Autodesk Fusion 360 part; units mm, degrees
sketch "Sketch1" plane through (0, 0, 0) normal (0, 0, 1) x (1, 0, 0)
  line L0 (33, 21) -> (-33, 21)
  line L1 (-33, 21) -> (-33, -21)
  line L2 (-33, -21) -> (33, -21)
  line L3 (33, -21) -> (33, 21)
  line L4 (33, 21) -> (-33, -21) construction
  line L5 (-33, 21) -> (33, -21) construction
  dimension "d1" = 66
  dimension "d2" = 42
extrude "Extrude1" add sketch "Sketch1" along normal blind 12
chamfer "Chamfer1" distance 12 angle 45 2 edges at (33, -21, 6) (33, 21, 6)
sketch "Sketch2" plane through (0, 0, 12) normal (0, 0, 1) x (-1, 0, 0)
  line L0 (-33, -9) -> (-21, -21)
  line L1 (-21, -21) -> (33, -21)
  line L2 (33, -21) -> (33, 21)
  line L3 (33, 21) -> (-21, 21)
  line L4 (-21, 21) -> (-33, 9)
  line L5 (-33, 9) -> (-33, -9)
  line L6 (33, -21) -> (21, -21)
  line L7 (21, -21) -> (21, 21)
  line L8 (21, 21) -> (33, 21)
  line L9 (33, 21) -> (33, -21)
  dimension "d6" = 12
extrude "Extrude2" add sketch "Sketch2" along normal blind 48 contours L1 L2 L3 L6 L7 L8 L9
fillet "Fillet1" radius 21 2 edges at (-27, 21, 60) (-27, -21, 60)
sketch "Sketch3" plane through (0, 0, 0) normal (0, 1, 0) x (1, 0, 0)
  line L0 (-20.8442, -53.799) -> (-20.8442, -11.799)
  line L1 (-20.8442, -11.799) -> (33.1558, -11.799)
  line L2 (33.1558, -11.799) -> (-20.8442, -53.799)
  dimension "d11" = 42
  dimension "d12" = 54
extrude "Extrude3" add sketch "Sketch3" along normal mid plane 12
equation "d7 = 60 mm - 12 mm"
equation "d12 = 66 mm - 12 mm"
Verification items for the finished model (mm, model axes). A direction names the side the tool comes from. Round coordinates to 2 decimals unless told otherwise and drop trailing zeros. Write each loop counter-clockwise with the first axis right and the second up, starting at its lowest first coordinate (ties: lowest second). Pieces come first, ordered by that corner, then holes.
(1) Depth check by flat-ended pin: pin 1 Ø10 at (y, z) = (11.5, 53.5) entering from +X; pin 2 Ø12.5 at (x, z) = (5, 26) entering from -Y; pin 3 Ø12.5 at (y, z) = (-7, 40.5) entering from +X. Enter the tip coordinate at first touch or a pass-through.
Returned:
pin 1: stops at x = -21
pin 2: stops at y = -6
pin 3: stops at x = 4.19
(2) Section check D-D (z = 28). Enter the section's corners in (x, y).
Returned:
outline: (-33, -21) - (-21, -21) - (-21, 21) - (-33, 21) - close; (-20.84, -6) - (12.33, -6) - (12.33, 6) - (-20.84, 6) - close
(3) Section check B-B (x = 28). Enter the section's corners in (y, z).
Returned:
outline: (-14, 0) - (14, 0) - (14, 12) - (6, 12) - (6, 15.81) - (-6, 15.81) - (-6, 12) - (-14, 12) - close
(4) Section check A-A (z = 17.5). Enter the section's corners in (x, y).
Returned:
outline: (-33, -21) - (-21, -21) - (-21, 21) - (-33, 21) - close; (-20.84, -6) - (25.83, -6) - (25.83, 6) - (-20.84, 6) - close
(5) Mould release check, pull along X, two halves, no side actions. Record for faces 3 (the flat face through (27, -15, 6)), 4 (the flat face through (-20.844, 0, 33)), 5 (the flat face through (0, 6, 28)), 6 (the flat face through (-21, 0, 36)): pulls with the +X half, pulls with the -X half, needs draft (parallel to the pull), parting line crosses it, or undercut.
Returned:
face 3: pulls with the +X half
face 4: undercut
face 5: needs draft
face 6: undercut
(6) Access from +Z, -Z, +X, -X, +Y, -Y to the whole of each face (thin tool, end or side, straight path). Record for faces 1 (the flat face through (0, -6, 28)), 2 (the flat face through (6.4, -0.08, 32.61)).
Returned:
face 1: +Z, +X, -Y
face 2: +Z, +X, +Y, -Y
(7) Section check C-C (y = -8). Enter the section's corners in (x, z).
Returned:
outline: (-33, 0) - (33, 0) - (33, 12) - (-21, 12) - (-21, 58.42) - (-33, 58.42) - close
(8) Material ranges on line 1 (X direction, y = 17.5, z = 50.5); line 2 (Y direction, x = 6, z = 24); line 3 (X direction, y = -3.5, z = 14.5), recorded low to high.
Returned:
line 1: x = -33 to -21
line 2: y = -6 to 6
line 3: x = -33 to -21, -20.84 to 29.68
